Could you check a few things on this model? Use its own coordinates, in mm. A direction names the side the tool comes from. Round coordinates to 2 decimals unless told otherwise and drop trailing zeros. Write each loop counter-clockwise with the first axis right and the second up, starting at its lowest first coordinate (ties: lowest second). Pieces come first, ordered by that corner, then holes. Notation, with made-up numbers: (88, 36.5) -> (126, 36.5) arc R12 ccw to (126, 51.5) -> close; hole circle Ø3 at (-1.5, 6). An arc over 180 degrees is marked (long way). Answer in a Markdown table with one row per item.
from build123d import *

# Parameters (mm, degrees)
F1_DEPTH = 9.525
F2_R     = 4.7625
F3_DEPTH = 9.526
F4_R     = 1.524
F5_DEPTH = 25.4
F6_R     = 2.54


with BuildPart() as f1:
    # F0 (on Front) → F1 (new body)
    with BuildSketch(Plane.XZ):
        Polygon((6.35, 12.7), (6.35, 31.75), (0, 31.75), (0, 0), (38.1, 0), (38.1, 12.7), align=None)
    extrude(amount=-F1_DEPTH)

    # F2 (on Front) → F3 (cut, through all)
    with BuildSketch(Plane.XZ):
        with Locations((31.75, 6.35)):
            Circle(F2_R)
    extrude(amount=-F3_DEPTH, mode=Mode.SUBTRACT)

    # F4 (on Right) → F5 (cut)
    with BuildSketch(Plane.YZ):
        with Locations((4.7625, 28.575)):
            Circle(F4_R)
        with Locations((4.7625, 18.575)):
            Circle(F4_R)
    extrude(amount=F5_DEPTH, mode=Mode.SUBTRACT)

    # F6
    f6_edges = [f1.edges().sort_by_distance(p)[0] for p in [
        (0, 4.7625, 0),
        (38.1, 4.7625, 0),
        (38.1, 4.7625, 12.7),
        (6.35, 4.7625, 12.7),
    ]]
    fillet(f6_edges, radius=F6_R)


solid = f1.part
1) Thinking about a two-plate mould opening in X: for faces 1 (the face through (36.293, 4.696, 7.781)), 2 (the face through (15, 9.525, 9)), 3 (the face through (0, 6, 17)), 4 (the face through (7.074, 4.829, 13.464)), which applies, +X half, -X half, draft (parallel to the pull), parting line (faces both ways), or undercut?
Findings:
| item | result |
|---|---|
| face 1 | undercut |
| face 2 | draft |
| face 3 | -X half |
| face 4 | +X half |
2) Imagine slicing it at A-A, the plane x = 31.75. Please give me the cut outline in (y, z) (1 decimal).
Findings:
| item | result |
|---|---|
| outline | (0, 0) -> (9.5, 0) -> (9.5, 1.6) -> (0, 1.6) -> close; (0, 11.1) -> (9.5, 11.1) -> (9.5, 12.7) -> (0, 12.7) -> close |
3) Please list where these lines run through material, in increasing order: line 1 (Z direction, x = 31.75, y = 5.5); line 2 (Z direction, x = 11, y = 4.25); line 3 (X direction, y = 0.5, z = 28).
Findings:
| item | result |
|---|---|
| line 1 | z = 0 to 1.59, 11.11 to 12.7 |
| line 2 | z = 0 to 12.7 |
| line 3 | x = 0 to 6.35 |
4) Imagine slicing it at D-D, the plane x = 4.5. Count the separate pieces of the cut face and the enclosed holes in it, plus the area to 3 significant figures.
Findings:
| item | result |
|---|---|
| separate pieces | 1 |
| enclosed holes | 2 |
| area | 288 mm^2 |
5) For pin 1 (3.5 mm diameter, centred on y = 4.76, z = 18.58, fed in from +X); pin 2 (1 mm diameter, centred on y = 4, z = 22, fed in from +X); pin 3 (3 mm diameter, centred on x = 23, y = 2.5, fed in from +Z), each with a flat end and sliding along its axis, tell me the tip position at first contact or that it passes through.
Findings:
| item | result |
|---|---|
| pin 1 | stops at x = 6.35 |
| pin 2 | stops at x = 6.35 |
| pin 3 | stops at z = 12.7 |
6) Imagine slicing it at B-B, the plane z = 6.35. Please give me the cut outline in (x, y) (1 decimal), plus the area to 3 significant figures.
Findings:
| item | result |
|---|---|
| outline | (0, 0) -> (27, 0) -> (27, 9.5) -> (0, 9.5) -> close; (36.5, 0) -> (38.1, 0) -> (38.1, 9.5) -> (36.5, 9.5) -> close |
| area | 272 mm^2 |
7) For faces 5 (the face through (6.35, 5, 23)), 6 (the face through (15, 0, 9)), which set-ups out of +Z, -Z, +X, -X, +Y, -Y let a thin tool reach every point of the face, with its end or its side?
Findings:
| item | result |
|---|---|
| face 5 | +Z, +X, +Y, -Y |
| face 6 | +Z, -Z, +X, -X, -Y |
